The listing builds one solid part. Answer for the finished solid, in the listing's coordinates (mm). Round coordinates to 2 decimals unless told otherwise and drop trailing zeros. Loops run counter-clockwise (first coordinate to the right, second up) from the corner with the lowest first, then second, coordinate; pieces in that order, holes last. Notation, with made-up numbers: (42.5, -11) - (66.5, -11) arc R21 ccw to (66.5, -2) - close; hole circle Ø5 at (-0.75, 32). An arc over 180 degrees is marked (long way). Write item = value, one per line. Start each with the question number.
1) Section B-B, the plane x = 16.5 is taken. Determine the outline of the cut face in (y, z).
2) Straight lines are drawn through the part: line 1 along Y through (x, z) = (-23.62, 0.7); line 2 along Y through (x, z) = (15.5, 0.1); line 3 along X through (y, z) = (24.5, 1). For each, find the intervals that lie inside material, in ascending order.
3) Section C-C, the plane y = 20.5 is taken. Determine the outline of the cut face in (x, z).
4) Given pin 1 Ø1.5 at (x, z) = (-21.5, 2) entering from +Y; pin 2 Ø2 at (x, y) = (16.38, 5.242) entering from +Z; pin 3 Ø1.5 at (x, z) = (-0.5, 2) entering from -Y, each flat-ended and moving along its own axis, determine where each tip first touches the part or whether it passes through.
5) Section D-D, the plane z = 1.65 is taken. Give the number of separate pieces and of enclosed holes in the cut face, and give its area (3 significant figures).
6) Section A-A, the plane x = -23.62 is taken. Determine the outline of the cut face in (y, z).
Autodesk Inventor part; units mm, degrees
ref_plane "YZ Plane" through (0, 0, 0) normal (1, 0, 0) x (0, 1, 0)
ref_plane "XZ Plane" through (0, 0, 0) normal (0, 1, 0) x (-1, 0, 0)
ref_plane "XY Plane" through (0, 0, 0) normal (0, 0, 1) x (1, 0, 0)
sketch "Szkic1" plane through (0, 0, 0) normal (0, 0, 1) x (1, 0, 0)
  circle A0 centre (-23.62, 45.242) radius 1.65
  circle A1 centre (16.38, 45.242) radius 1.65
  circle A2 centre (-23.62, 5.242) radius 1.65
  circle A3 centre (16.38, 5.242) radius 1.65
  circle A4 centre (-3.62, 25.242) radius 24
  arc A5 (-18.8305, 43.8065) -> (-22.1845, 40.4524) centre (-23.62, 45.242) ccw
  arc A6 (-22.1845, 10.0315) -> (-18.8305, 6.6774) centre (-23.62, 5.242) ccw
  arc A7 (14.9445, 40.4524) -> (11.5905, 43.8065) centre (16.38, 45.242) ccw
  arc A8 (11.5905, 6.6774) -> (14.9445, 10.0315) centre (16.38, 5.242) ccw
  point P0 (0, 0)
  point P1 (0, 0)
  dimension "d10" = 3.3
  dimension "d11" = 3.3
  dimension "d12" = 3.3
  dimension "d15" = 10
  dimension "d16" = 10
  dimension "d17" = 10
  dimension "d18" = 10
  dimension "d22" = 3.3
extrude "Wyciągnięcie proste1" add sketch "Szkic1" along normal blind 2.5
fillet "Zaokrąglenie1" radius 3 8 edges at (-22.1845, 10.0315, 1.25) (-18.8305, 6.6774, 1.25) (14.9445, 10.0315, 1.25) (11.5905, 6.6774, 1.25) (11.5905, 43.8065, 1.25) (14.9445, 40.4524, 1.25) (-18.8305, 43.8065, 1.25) (-22.1845, 40.4524, 1.25)
equation "\"d10\" = d12"
equation "\"d11\" = d12"
equation "\"d22\" = d12"
properties part number "3DP_ABS_Electronics_Colling_Fan_Grill_Honeycomb" material "Aluminium 5005-H12"
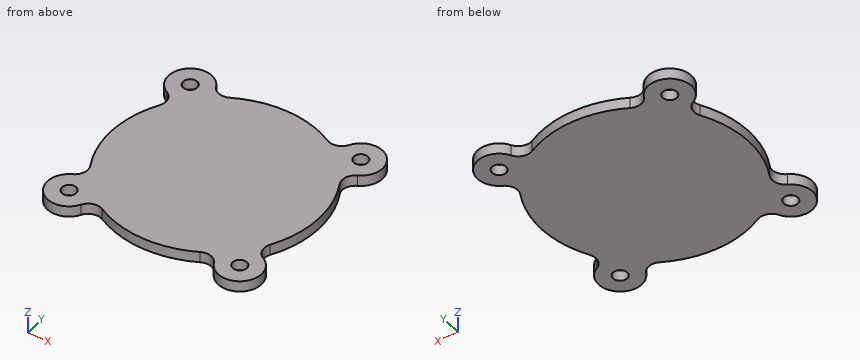
Geometry check:
q1.outline = (0.24, 0) - (3.6, 0) - (3.6, 2.5) - (0.24, 2.5) - close; (6.89, 0) - (43.6, 0) - (43.6, 2.5) - (6.89, 2.5) - close; (46.89, 0) - (50.24, 0) - (50.24, 2.5) - (46.89, 2.5) - close
q2.line_1 = 0.24 to 3.59, 6.89 to 43.59, 46.89 to 50.24
q2.line_2 = 0.32 to 3.85, 6.64 to 43.85, 46.64 to 50.16
q2.line_3 = -27.61 to 20.37
q3.outline = (-27.15, 0) - (19.91, 0) - (19.91, 2.5) - (-27.15, 2.5) - close
q4.pin_1 = 50.05
q4.pin_2 = through
q4.pin_3 = 1.36
q5.separate_pieces = 1
q5.enclosed_holes = 4
q5.area = 2,110 mm2
q6.outline = (0.24, 0) - (3.59, 0) - (3.59, 2.5) - (0.24, 2.5) - close; (6.89, 0) - (43.59, 0) - (43.59, 2.5) - (6.89, 2.5) - close; (46.89, 0) - (50.24, 0) - (50.24, 2.5) - (46.89, 2.5) - close
